Source: CAD feature listing. Evaluate the final solid. Frame: model axes, mm. Face numbers are marked on the shaded views. A direction names the side the tool comes from. Coordinates: 2 decimals unless noted, no trailing zeros. Order: outer loops, then holes, each group sorted by start corner. A loop starts at its lowest first (then second) coordinate and runs counter-clockwise, first axis right, second up.
```python
from build123d import *

# Parameters (mm, degrees)
F1_W     = 38.1
F1_H     = 38.1
F2_DEPTH = 19.05
F3_R     = 19.05
F4_DEPTH = 30.226
F5_W     = 11.2522
F5_H     = 11.7586595006
F6_DEPTH = 68.327


# Not quite as in the source:
# - a variable given as a bare number and used for a length is read in inches; the dataset says mm whatever the document's units were


with BuildPart() as f2:
    # F1 (on Front) → F2 (new body, symmetric)
    with BuildSketch(Plane.XZ):
        Rectangle(F1_W, F1_H)
    extrude(amount=F2_DEPTH, both=True)

    # F3 (on face) → F4 (join)
    with BuildSketch(Plane.YZ.offset(19.05)):
        Circle(F3_R)
    extrude(amount=F4_DEPTH)

    # F5 (on face) → F6 (cut, through all)
    with BuildSketch(Plane.YZ.offset(49.276)):
        with Locations((2.8142485544, 7.924313657)):
            Rectangle(F5_W, F5_H)
    extrude(amount=-F6_DEPTH, mode=Mode.SUBTRACT)


solid = f2.part
```
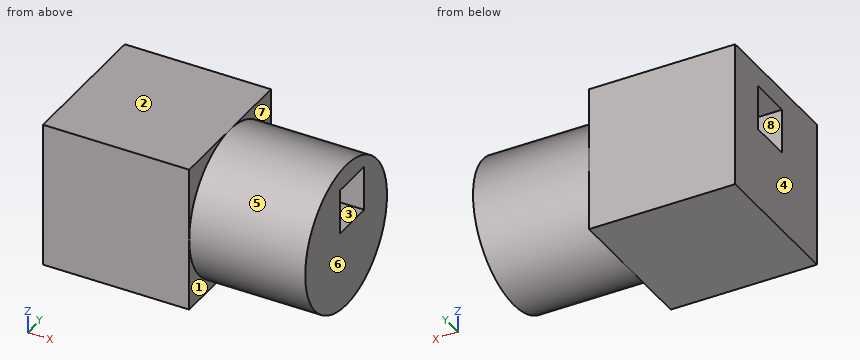
1. Section query B-B on z = 9. Return loops of the section in (x, y).
Findings:
outline: (-19.05, -19.05) - (19.05, -19.05) - (19.05, -16.79) - (49.28, -16.79) - (49.28, -2.81) - (-19.05, -2.81) - close; (-19.05, 8.44) - (49.28, 8.44) - (49.28, 16.79) - (19.05, 16.79) - (19.05, 19.05) - (-19.05, 19.05) - close
2. Pin query (flat end, axial travel): P1, Ø3, axis at x = 34, z = 5, coming from the +Y side; P2, Ø21, axis at y = 13.5, z = 13.5, coming from the +X side; P3, Ø6, axis at x = 28, z = 9.5, coming from the -Y side. Return the tip coordinate at first contact, or that it passes through.
Findings:
P1: stops at y = 18.73
P2: stops at x = 49.28
P3: stops at y = -17.91
3. Ray query, line 1 (Y direction, x = -16, z = 3); line 2 (Z direction, x = 41, y = -2); line 3 (Z direction, x = 33.5, y = 1). Return the intervals inside material, ascending.
Findings:
line 1: y = -19.05 to -2.81, 8.44 to 19.05
line 2: z = -18.94 to 2.04, 13.8 to 18.94
line 3: z = -19.02 to 2.04, 13.8 to 19.02
4. Section query C-C on y = -1.5. Return loops of the section in (x, z).
Findings:
outline: (-19.05, -19.05) - (19.05, -19.05) - (19.05, -18.99) - (49.28, -18.99) - (49.28, 2.04) - (-19.05, 2.04) - close; (-19.05, 13.8) - (49.28, 13.8) - (49.28, 18.99) - (19.05, 18.99) - (19.05, 19.05) - (-19.05, 19.05) - close
5. Section query A-A on x = -1.5. Return loops of the section in (y, z), plus the area to 3 significant figures.
Findings:
outline: (-19.05, -19.05) - (19.05, -19.05) - (19.05, 19.05) - (-19.05, 19.05) - close; hole (-2.81, 2.04) - (8.44, 2.04) - (8.44, 13.8) - (-2.81, 13.8) - close
area: 1,320 mm2
6. Section query D-D on y = -10. Return loops of the section in (x, z).
Findings:
outline: (-19.05, -19.05) - (19.05, -19.05) - (19.05, -16.21) - (49.28, -16.21) - (49.28, 16.21) - (19.05, 16.21) - (19.05, 19.05) - (-19.05, 19.05) - close
7. Access query for the marked faces 4, 5, 6, 7 and 8. Directions: +Z, -Z, +X, -X, +Y, -Y. A direction counts if a zero-diameter tool reaches every point of the face in a straight line with its end or side. Return the directions, or none.
Findings:
face 4: +Z, -Z, -X, +Y, -Y
face 5: +X
face 6: +Z, -Z, +X, +Y, -Y
face 7: +Z, +X, +Y
face 8: +X, -X
8. Draft query along Z for the marked faces 1, 2 and 3. Return one class per face: released by +Z, released by -Z, zero draft, split by the parting line, or undercut.
Findings:
face 1: zero draft
face 2: released by +Z
face 3: undercut
